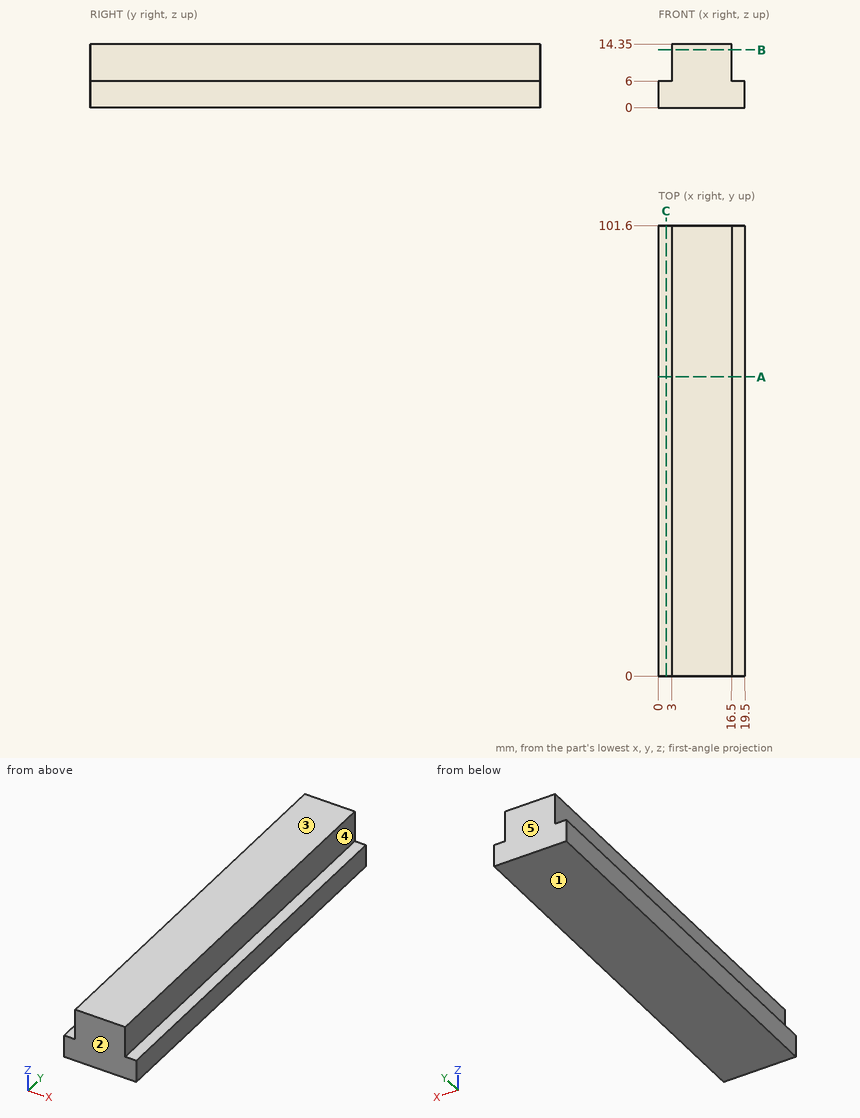
Source: three-view drawing plus pictorial views. Frame: mm from the lowest corner of the part. A direction names the side the tool comes from. Give positions to 0.01 mm unless a question says otherwise; leave off trailing zeros. Write each loop counter-clockwise with the first axis right and the second up, starting at its lowest first coordinate (ties: lowest second). Pieces come first, ordered by that corner, then holes. Notation, with made-up numbers: M -37.5,86.25 L -16.5,86.25 A15 cw -16.5,108.25 Z; hole C -18.5,14 d1. An arc over 180 degrees is marked long. Use one line per item in the form item = value.
1. Reachability of the marked faces 4 and 5 from +Z, -Z, +X, -X, +Y, -Y: full face, straight path, thin tool, end or side. Return the list, or none.
Outcome:
face_4 = +Z, +X, +Y, -Y
face_5 = +Z, -Z, +X, -X, +Y
2. Cut plane A-A on y = 67.5. Return loops of the section in (x, z).
Outcome:
outline = M 0,0 L 19.5,0 L 19.5,6 L 16.5,6 L 16.5,14.35 L 3,14.35 L 3,6 L 0,6 Z
3. Cut plane C-C on x = 1.75. Return loops of the section in (y, z).
Outcome:
outline = M 0,0 L 101.6,0 L 101.6,6 L 0,6 Z
4. Cut plane B-B on z = 13. Return loops of the section in (x, y).
Outcome:
outline = M 3,0 L 16.5,0 L 16.5,101.6 L 3,101.6 Z
5. Ray query, L1, parallel to X at y = 24, z = 13.75; L2, parallel to Z at x = 17, y = 94.5. Return the intervals inside material, ascending.
Outcome:
L1 = 3 to 16.5
L2 = 0 to 6
6. First-contact query: P1, Ø0.9, axis at x = 18.5, y = 76, coming from the +Z side. Flat tip, straight axial feed; report the tip coordinate or a pass-through.
Outcome:
P1 = 6
7. Mould query, pull axis Z, two halves, no side actions, for the marked faces 1, 2 and 3. Classes: released by +Z, released by -Z, zero draft, split by the parting line, or undercut.
Outcome:
face_1 = released by -Z
face_2 = zero draft
face_3 = released by +Z
